Here's the drawing with two shaded views (mm, measured from the low corner). I have some questions. A direction names the side the tool comes from. Round coordinates to 2 decimals unless told otherwise and drop trailing zeros. Loops run counter-clockwise (first coordinate to the right, second up) from the corner with the lowest first, then second, coordinate; pieces in that order, holes last. Notation, with made-up numbers: M 24.5,-38.5 L 35.5,-38.5 A18 ccw 35.5,-11.5 Z; hole C 83.25,8 d2. An arc over 180 degrees is marked long. Answer as CSV lines item,"result".
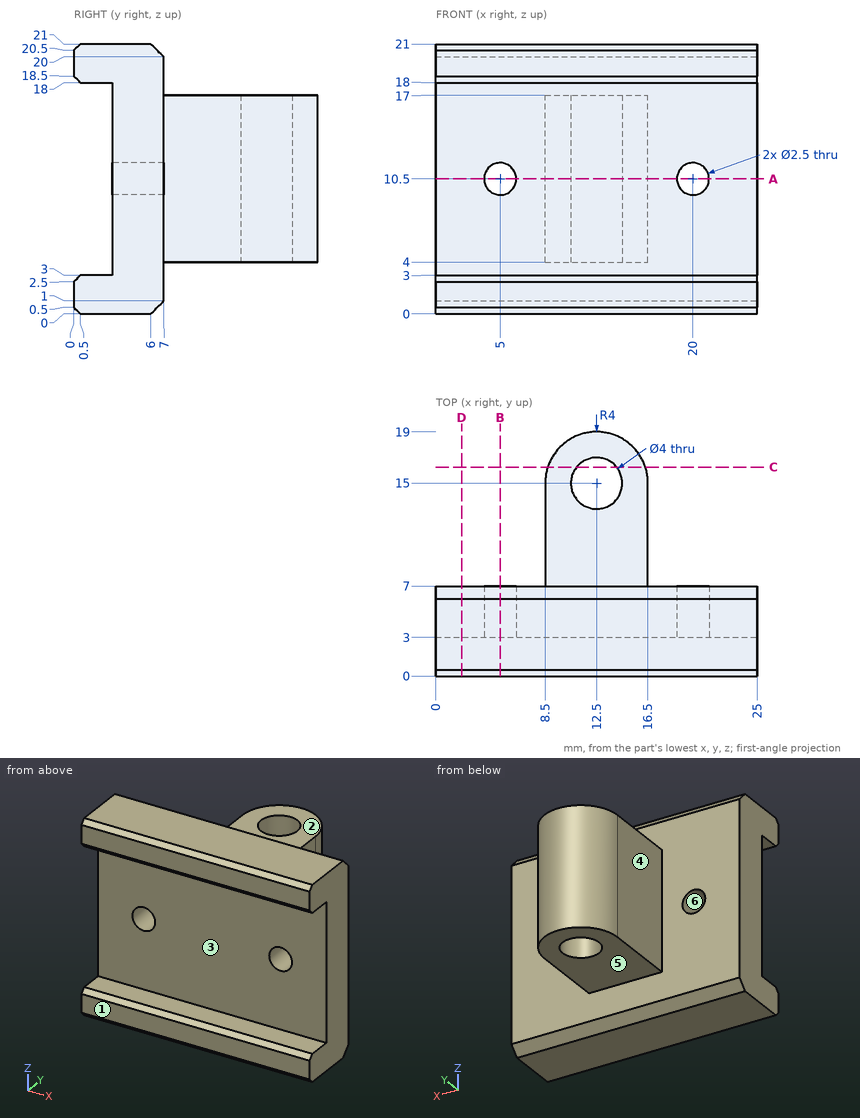
1. Which directions (+Z, -Z, +X, -X, +Y, -Y) give clear straight access to the entire face, cutting with the end or side of a thin tool? Please do the marked faces 1, 2 and 3.
Evaluation:
face 1,"+Z, -Z, +X, -X, -Y"
face 2,"+Z, +X, -X, +Y"
face 3,"+X, -X, -Y"
2. I want a section at D-D, the plane x = 2. Please give me the cut outline in (y, z), and give its area (4 significant figures).
Evaluation:
outline,"M 0,0.5 L 0.5,0 L 6,0 L 7,1 L 7,20 L 6,21 L 0.5,21 L 0,20.5 L 0,18.5 L 0.5,18 L 3,18 L 3,3 L 0.5,3 L 0,2.5 Z"
area,"100.5 mm²"
3. I want a section at C-C, the plane y = 16.25. Please give me the cut outline in (x, z), and give its area (3 significant figures).
Evaluation:
outline,"M 8.7,4 L 10.94,4 L 10.94,17 L 8.7,17 Z; M 14.06,4 L 16.3,4 L 16.3,17 L 14.06,17 Z"
area,"58.2 mm²"
4. If I drill on line 1 (X direction, y = 5.8, z = 10.5); line 2 (Z direction, x = 23.25, y = 2.5); line 3 (Y direction, x = 12.5, z = 7), over which ranges is the centre line in solid material (lowest first)? Write a range as [from, to].
Evaluation:
line 1,"x = [0, 3.75], [6.25, 18.75], [21.25, 25]"
line 2,"z = [0, 3], [18, 21]"
line 3,"y = [3, 13], [17, 19]"
5. For P1, Ø8, axis at y = 15.5, z = 3.5, coming from the +X side; P2, Ø10, axis at x = 4.5, y = 13.5, coming from the +Z side; P3, Ø4, axis at y = 12, z = 12, coming from the -X side; P4, Ø6.5, axis at y = 10, z = 9, coming from the +X side, each with a flat end and sliding along its axis, tell me the tip position at first contact or that it passes through.
Evaluation:
P1,"stops at x = 16.5"
P2,"stops at z = 17"
P3,"stops at x = 8.5"
P4,"stops at x = 25"
6. We'd pull the mould along X, two halves only. Please class the marked faces 4, 5 and 6: pulls with the +X half, pulls with the -X half, needs draft (parallel to the pull), parting line crosses it, or undercut.
Evaluation:
face 4,"pulls with the -X half"
face 5,"needs draft"
face 6,"undercut"
7. I want a section at B-B, the plane x = 5. Please give me the cut outline in (y, z).
Evaluation:
outline,"M 0,0.5 L 0.5,0 L 6,0 L 7,1 L 7,9.25 L 3,9.25 L 3,3 L 0.5,3 L 0,2.5 Z; M 0,18.5 L 0.5,18 L 3,18 L 3,11.75 L 7,11.75 L 7,20 L 6,21 L 0.5,21 L 0,20.5 Z"
8. I want a section at A-A, the plane z = 10.5. Please give me the cut outline in (x, y), and give its area (3 significant figures).
Evaluation:
outline,"M 0,3 L 3.75,3 L 3.75,7 L 0,7 Z; M 6.25,3 L 18.75,3 L 18.75,7 L 16.5,7 L 16.5,15 A4 ccw 8.5,15 L 8.5,7 L 6.25,7 Z; M 21.25,3 L 25,3 L 25,7 L 21.25,7 Z; hole C 12.5,15 d4"
area,"157 mm²"
